Design review of the part shown in the three views and the two pictorial views. Dimensions are in mm from the part's minimum x, y and z. Coordinates: 2 decimals unless noted, no trailing zeros. Write each loop counter-clockwise with the first axis right and the second up, starting at its lowest first coordinate (ties: lowest second). Pieces come first, ordered by that corner, then holes.
Q1. Take a section at B-B, the plane x = 2.25. Write out the cut boundary in (y, z).
Q2. Take a section at C-C, the plane y = 14. Write out the cut boundary in (x, z).
Q3. Take a section at A-A, the plane y = 80.5. Write out the cut boundary in (x, z), plus the area to 3 significant figures.
Q4. Take a section at D-D, the plane z = 123.5. Write out the cut boundary in (x, y).
Q5. For L1, parallel to Z at x = 2, y = 93; L2, parallel to Z at x = 2.5, y = 23; L3, parallel to Y at x = 2, z = 42, list the stretches that pass through material, from the lowest coordinate up.
Q6. For pin 1 Ø1.9 at (x, y) = (4.5, 32) entering from -Z; pin 2 Ø1.9 at (x, y) = (3.5, 86.5) entering from -Z; pin 3 Ø1 at (x, y) = (5, 76) entering from +Z; pin 4 Ø1.9 at (x, z) = (2, 11) entering from +Y, all flat-tipped, find the tip position at first contact; note any pin that passes through.
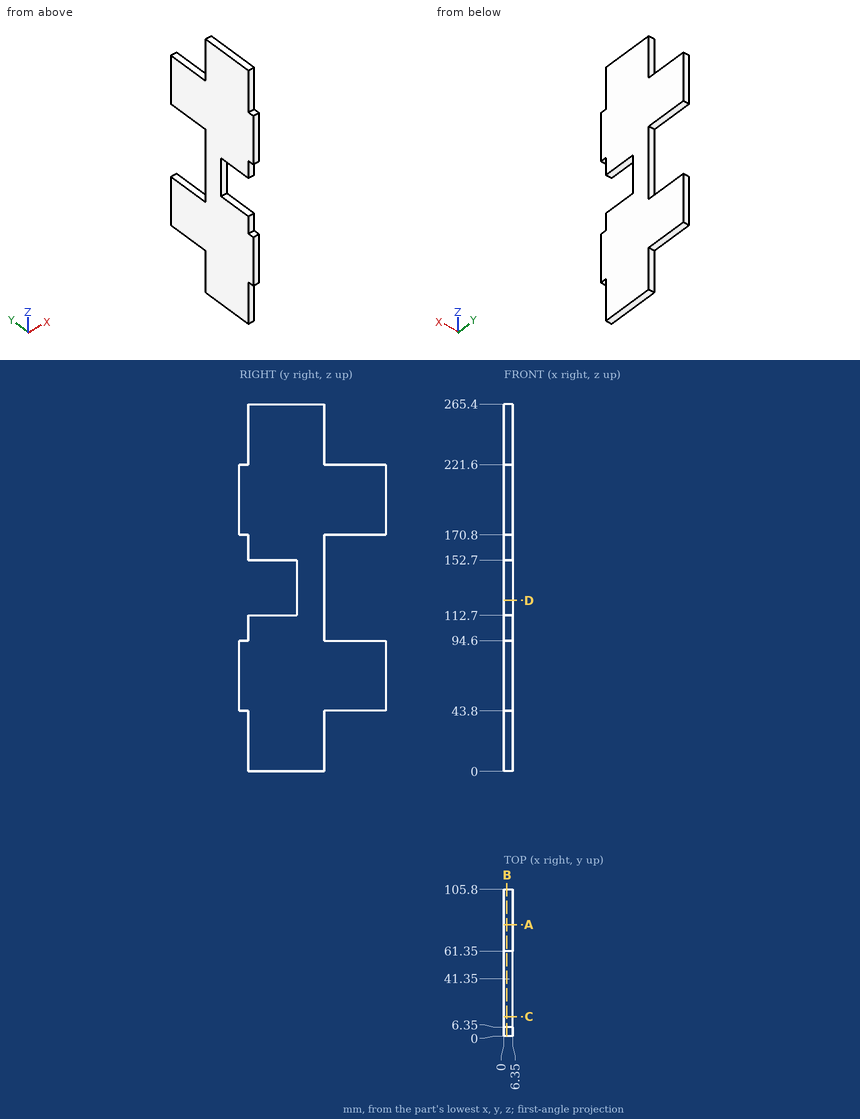
Responses:
1. outline: (0, 43.8) - (6.35, 43.8) - (6.35, 0) - (61.35, 0) - (61.35, 43.8) - (105.8, 43.8) - (105.8, 94.6) - (61.35, 94.6) - (61.35, 170.8) - (105.8, 170.8) - (105.8, 221.6) - (61.35, 221.6) - (61.35, 265.4) - (6.35, 265.4) - (6.35, 221.6) - (0, 221.6) - (0, 170.8) - (6.35, 170.8) - (6.35, 152.7) - (41.35, 152.7) - (41.35, 112.7) - (6.35, 112.7) - (6.35, 94.6) - (0, 94.6) - close
2. outline: (0, 0) - (6.35, 0) - (6.35, 112.7) - (0, 112.7) - close; (0, 152.7) - (6.35, 152.7) - (6.35, 265.4) - (0, 265.4) - close
3. outline: (0, 43.8) - (6.35, 43.8) - (6.35, 94.6) - (0, 94.6) - close; (0, 170.8) - (6.35, 170.8) - (6.35, 221.6) - (0, 221.6) - close
3. area: 645 mm2
4. outline: (0, 41.35) - (6.35, 41.35) - (6.35, 61.35) - (0, 61.35) - close
5. L1: z = 43.8 to 94.6, 170.8 to 221.6
5. L2: z = 0 to 112.7, 152.7 to 265.4
5. L3: y = 6.35 to 61.35
6. pin 1: stops at z = 0
6. pin 2: stops at z = 43.8
6. pin 3: stops at z = 221.6
6. pin 4: stops at y = 61.35
